Here's how the part is built. I have some questions about the finished solid (model axes, mm). Face numbers are marked on the shaded views. A direction names the side the tool comes from. Give positions to 0.01 mm unless a question says otherwise; leave off trailing zeros. Loops run counter-clockwise (first coordinate to the right, second up) from the corner with the lowest first, then second, coordinate; pieces in that order, holes last.
Q1. Will these pins go through, and if not, where does the flat tip stop? P1, Ø2, axis at x = 5, z = 5, coming from the -Y side; P2, Ø1.5, axis at x = 3, y = 2, coming from the +Z side; P3, Ø2, axis at y = 4.5, z = 10.5, coming from the +X side.
Q2. If we section it at A-A (z = 4.5): Please give me the cut outline in (x, y).
Q3. If we section it at C-C (z = 2): Please give me the cut outline in (x, y).
Q4. If we section it at D-D (x = 6.5): Please give me the cut outline in (y, z), plus the area to 3 significant figures.
Q5. I need wall thicknesses on line 1 (Z direction, x = 5, y = 3.6); line 2 (Z direction, x = 4, y = 0.85); line 3 (Y direction, x = 2.5, z = 2.2). Which ranges of each line are inside material? Lowest first, please.
Q6. For the marked faces 5, 6 and 7, which set-ups out of +Z, -Z, +X, -X, +Y, -Y let a thin tool reach every point of the face, with its end or its side?
Q7. We'd pull the mould along X, two halves only. Please class the marked faces 1, 2, 3 and 4: +X half, -X half, draft (parallel to the pull), parting line (faces both ways), or undercut.
Q8. If we section it at B-B (y = 3.85): Please give me the cut outline in (x, z) (3 decimals), plus the area to 3 significant figures.
Autodesk Inventor part; units mm, degrees
ref_plane "YZ Plane" through (0, 0, 0) normal (1, 0, 0) x (0, 1, 0)
ref_plane "XZ Plane" through (0, 0, 0) normal (0, 1, 0) x (-1, 0, 0)
ref_plane "XY Plane" through (0, 0, 0) normal (0, 0, 1) x (1, 0, 0)
sketch "スケッチ1" plane through (0, 0, 0) normal (0, 1, 0) x (-1, 0, 0)
  line L0 (0, 0) -> (-5, 0)
  line L1 (-5, 0) -> (-5, 5)
  line L2 (-5, 5) -> (0, 5)
  line L3 (0, 5) -> (0, 0)
  circle A0 centre (-5, 5) radius 1.25
  line L4 (0, 0) -> (0, 15)
  circle A1 centre (-5, 5) radius 5
  circle A2 centre (-5, 5) radius 3
  line L5 (-8, 5) -> (-8, 0)
  line L6 (-8, 0) -> (-8, 15)
  line L7 (-8, 15) -> (0, 15)
  line L8 (-5, 5) -> (-5, 15)
  line L9 (-5, 10) -> (-8, 10)
  circle A3 centre (-5, 5) radius 2.25
  circle A4 centre (-5, 10) radius 2.5
  circle A5 centre (-5, 10) radius 4.5
  line L10 (-5, 10) -> (-0.9814, 7.975)
  line L11 (-5, 10) -> (-2.3337, 6.375)
  line L12 (-9.5, 10) -> (-10, 5)
  line L13 (-2.3337, 6.375) -> (-5, 10)
  line L14 (-5, 10) -> (-0.2269, 3.5108)
  line L15 (-0.2269, 3.5108) -> (-5, 0)
  line L16 (-2.3337, 6.375) -> (0, 5)
  point P0 (-3.5187, 7.9861)
  point P1 (-2.7674, 8.875)
  dimension "d0" = 5
  dimension "d1" = 5
  dimension "d2" = 2.5
  dimension "d3" = 15
  dimension "d4" = 6
  dimension "d5" = 4.5
  dimension "d8" = 5
  dimension "d10" = 9
extrude "押し出し1" add sketch "スケッチ1" along normal blind 5 contours L0 A1 L3 | A1 L5 A2 L1 | L15 A1 | L1 A2 L2 L14 L15 | A1 L14 L2 | L2 L14 L16 | A2 A5 A3 L1 | L1 A3 L2 A2 | A1 L12 A5 L6 L5 | L2 A2 L14 | L10 A4 A1 | A1 A4 L8 A5 | A2 L2 A3 A5 | A5 A3 L8 A4 A2 L11 | A3 A5 A0 L1 | L1 A0 L2 A3 | L6 A5 A2 | A2 A4 L11 | A5 A0 L8 A3 | A3 L2 A0 A5 | A5 A2 A4 L8 A3 | A3 L8 A0 A5 | A5 L6 A1 A4 A2 | A5 A1 L6 | L12 A5 A1 | L8 A4 L9 L6 A5 | L6 L9 A4 A1 | A1 A5 L6 picked at (-1.7314, 8.4555)
sketch "スケッチ3" plane through (5, 0, 0) normal (0, 0, -1) x (-1, 0, 0)
  line L0 (5, 0) -> (5, 5)
  line L1 (5, 0) -> (2.5, 0)
  line L2 (2.5, 0) -> (2.5, 2.5)
  line L3 (2.5, 2.5) -> (5, 2.5)
  line L4 (5, 2.5) -> (5, 0)
  circle A0 centre (2.5, 2.5) radius 1.55
  dimension "d13" = 2.5
  dimension "d14" = 2.5
  dimension "d15" = 3.1
extrude "押し出し2" cut sketch "スケッチ3" against normal blind 5 contours A0 L2 L3 | L3 L2 A0
properties part number "rod_exp1.1"
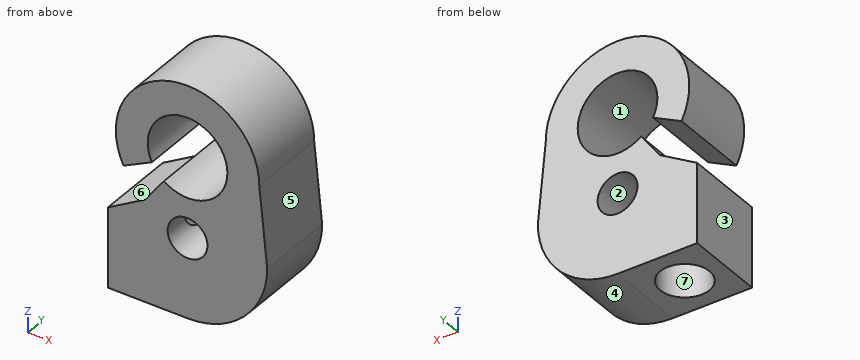
Check sheet entries:
1. P1: passes through
1. P2: stops at z = 14.32
1. P3: stops at x = 9.55
2. outline: (0, 0) - (3.85, 0) - (3.85, 1.75) arc R1.55 cw (long way) to (3.85, 3.25) - (3.85, 5) - (0, 5) - close; (6.15, 0) - (9.97, 0) - (9.97, 5) - (6.15, 5) - close
3. outline: (0, 0) - (9, 0) - (9, 5) - (0, 5) - close; hole circle Ø3.1 at (2.5, 2.5)
4. outline: (0, 0.23) - (5, 0.23) - (5, 8) - (0, 8) - close; (0, 12) - (5, 12) - (5, 14.24) - (0, 14.24) - close
4. area: 50.1 mm2
5. line 1: z = 0 to 3.75, 6.25 to 7.5, 12.5 to 14.5
5. line 2: z = 0 to 4.25, 5.75 to 7.71, 12.29 to 14.39
5. line 3: y = 0 to 0.95, 4.05 to 5
6. face 5: +Z, +X, +Y, -Y
6. face 6: -X, +Y, -Y
6. face 7: -Z
7. face 1: undercut
7. face 2: undercut
7. face 3: -X half
7. face 4: +X half
8. outline: (0, 0) - (1.738, 0) - (1.738, 5) - (3.262, 5) - (3.262, 0) - (5, 0) arc R5 ccw to (10, 5) - (9.5, 10) arc R4.5 ccw (long way) to (0.981, 7.975) - (2.767, 8.875) arc R2.5 cw (long way) to (3.519, 7.986) - (2.334, 6.375) - (0, 5) - close; hole circle Ø2.5 at (5, 5)
8. area: 84.3 mm2
